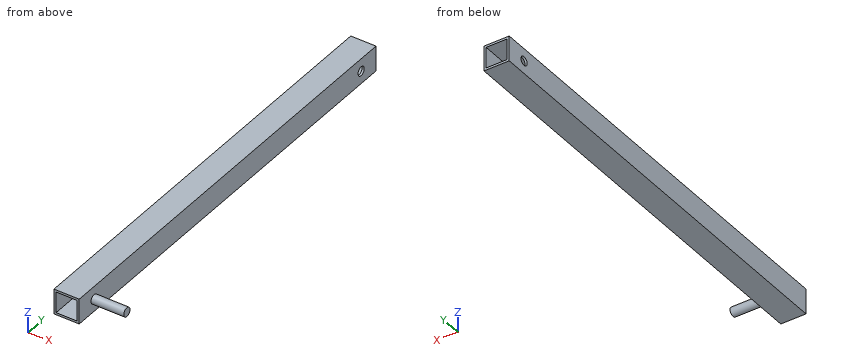
```python
from build123d import *

# Parameters (mm, degrees)
F0_W     = 35
F0_H     = 35
F0_W_2   = 29
F0_H_2   = 29
F1_DEPTH = 300
F2_R     = 6.25
F3_DEPTH = 35.56
F4_DEPTH = 80.518


with BuildPart() as f1:
    # F0 (on Front) → F1 (new body, symmetric)
    with BuildSketch(Plane.XZ):
        with Locations((-53.6115857959, -24.8530973494)):
            Rectangle(F0_W, F0_H)
        with Locations((-53.6115857959, -24.8530973494)):
            Rectangle(F0_W_2, F0_H_2, mode=Mode.SUBTRACT)
    extrude(amount=F1_DEPTH, both=True)

    # F2 (on face) → F3 (cut)
    with BuildSketch(Plane(origin=(-71.1115857959, 0, 0), x_dir=(0, -1, 0), z_dir=(-1, 0, 0))):
        with Locations((-270, -24.8530973494)):
            Circle(F2_R)
    extrude(amount=-F3_DEPTH, mode=Mode.SUBTRACT)

    # F2 (on face) → F4 (join)
    with BuildSketch(Plane(origin=(-71.1115857959, 0, 0), x_dir=(0, -1, 0), z_dir=(-1, 0, 0))):
        with Locations((270, -24.8530973494)):
            Circle(F2_R)
    extrude(amount=-F4_DEPTH)


solid = f1.part
```
Here's how the part is built. I have some questions about the finished solid (model axes, mm). Give positions to 0.01 mm unless a question says otherwise; leave off trailing zeros. Order: outer loops, then holes, each group sorted by start corner. A loop starts at its lowest first (then second) coordinate and runs counter-clockwise, first axis right, second up. Notation, with made-up numbers: M -35,11.5 L -6,11.5 A10 cw -6,27.5 Z; hole C 46.25,-16.5 d4. An arc over 180 degrees is marked long. Use a Markdown table: item, result. Add a question column.
1. I need wall thicknesses on probe 1 along X at (y, z) = (84.5, -33); probe 2 along Z at (x, y) = (-39.5, 171); probe 3 along Z at (x, y) = (-69, 270). Which ranges of each line are inside material? Lowest first, please. Write a range as from..to.
2. Suppose I cut it at B-B (x = -56.5). List the corners of the cut face in (y, z) for me.
3. Suppose I cut it at D-D (y = 83.5). List the corners of the cut face in (x, z) for me.
4. Suppose I cut it at A-A (y = 270). List the corners of the cut face in (x, z) for me.
5. Suppose I cut it at C-C (y = -270). List the corners of the cut face in (x, z) for me.
6. For pin 1 Ø8.5 at (y, z) = (86.5, -24) entering from +X, with a flat end and sliding along its axis, tell me the tip position at first contact or that it passes through.
Results list:
| question | item | result |
|---|---|---|
| 1 | probe 1 | x = -71.11..-68.11, -39.11..-36.11 |
| 1 | probe 2 | z = -42.35..-39.35, -10.35..-7.35 |
| 1 | probe 3 | z = -42.35..-31.1, -18.6..-7.35 |
| 2 | outline | M -300,-42.35 L 300,-42.35 L 300,-39.35 L -300,-39.35 Z; M -300,-10.35 L 300,-10.35 L 300,-7.35 L -300,-7.35 Z; C -270,-24.85 d12.5 |
| 3 | outline | M -71.11,-42.35 L -36.11,-42.35 L -36.11,-7.35 L -71.11,-7.35 Z; hole M -68.11,-39.35 L -39.11,-39.35 L -39.11,-10.35 L -68.11,-10.35 Z |
| 4 | outline | M -71.11,-42.35 L -36.11,-42.35 L -36.11,-31.1 L -39.11,-31.1 L -39.11,-39.35 L -68.11,-39.35 L -68.11,-31.1 L -71.11,-31.1 Z; M -71.11,-18.6 L -68.11,-18.6 L -68.11,-10.35 L -39.11,-10.35 L -39.11,-18.6 L -36.11,-18.6 L -36.11,-7.35 L -71.11,-7.35 Z |
| 5 | outline | M -71.11,-42.35 L -36.11,-42.35 L -36.11,-31.1 L 9.41,-31.1 L 9.41,-18.6 L -36.11,-18.6 L -36.11,-7.35 L -71.11,-7.35 Z; hole M -68.11,-39.35 L -39.11,-39.35 L -39.11,-31.1 L -68.11,-31.1 Z; hole M -68.11,-18.6 L -39.11,-18.6 L -39.11,-10.35 L -68.11,-10.35 Z |
| 6 | pin 1 | stops at x = -36.11 |
